from build123d import *

# Parameters (mm, degrees)
SKETCH1_R                  = 34.671
BOSS_EXTRUDE1_DEPTH        = 9.525
FILLET1_R                  = 5.08
SKETCH2_R                  = 4.0005
CUT_EXTRUDE1_DEPTH         = 5.08
F_10_CLEARANCE_HOLE1_D     = 5.1054
F_10_CLEARANCE_HOLE1_DEPTH = 4.445


with BuildPart() as part:
    # Sketch1 → Boss-Extrude1 (new body)
    with BuildSketch(Plane.XY):
        with Locations(Location((0, 0, 0), (0, 0, 180))):
            Circle(SKETCH1_R)
        with BuildLine():
            ThreePointArc((19.058413969, -22.135965238), (29.21, 0), (19.058413969, 22.135965238))
            ThreePointArc((19.058413969, 22.135965238), (11.8745, 20.567237314), (9.641101249, 27.573053271))
            ThreePointArc((9.641101249, 27.573053271), (-14.605, 25.296602045), (-28.699515217, 5.437088034))
            ThreePointArc((-28.699515217, 5.437088034), (-23.749, 0), (-28.699515217, -5.437088034))
            ThreePointArc((-28.699515217, -5.437088034), (-14.605, -25.296602045), (9.641101249, -27.573053271))
            ThreePointArc((9.641101249, -27.573053271), (11.8745, -20.567237314), (19.058413969, -22.135965238))
        make_face(mode=Mode.SUBTRACT)
    extrude(amount=BOSS_EXTRUDE1_DEPTH)

    # Fillet1
    fillet1_edges = [part.edges().sort_by_distance(p)[0] for p in [
        (-28.699515217, 5.437088034, 4.7625),
        (-28.699515217, -5.437088034, 4.7625),
        (9.641101249, -27.573053271, 4.7625),
        (19.058413969, -22.135965238, 4.7625),
        (19.058413969, 22.135965238, 4.7625),
        (9.641101249, 27.573053271, 4.7625),
    ]]
    fillet(fillet1_edges, radius=FILLET1_R)

    # Sketch2 → Cut-Extrude1 (cut)
    with BuildSketch(Plane(origin=(0, 0, 0), x_dir=(-1, 0, 0), z_dir=(0, 0, -1))):
        with Locations((-14.605, 25.296602045)):
            Circle(SKETCH2_R)
        with Locations((29.21, 0)):
            Circle(SKETCH2_R)
        with Locations((-14.605, -25.296602045)):
            Circle(SKETCH2_R)
    extrude(amount=-CUT_EXTRUDE1_DEPTH, mode=Mode.SUBTRACT)

    # #10 Clearance Hole1
    with Locations(Plane(origin=(0, 0, 5.08), x_dir=(-1, 0, 0), z_dir=(0, 0, -1))):
        with Locations((-14.605, 25.296602045), (29.21, 0), (-14.605, -25.296602045), (0, 0)):
            Hole(F_10_CLEARANCE_HOLE1_D / 2, depth=F_10_CLEARANCE_HOLE1_DEPTH)


solid = part.part
Work out the finished part from the listing and answer in its coordinate system (mm). A direction names the side the tool comes from. Coordinates: 2 decimals unless noted, no trailing zeros. Write each loop counter-clockwise with the first axis right and the second up, starting at its lowest first coordinate (ties: lowest second). Pieces come first, ordered by that corner, then holes. Notation, with made-up numbers: M 75,16 L 131,16 A21 cw 131,24 Z; hole C 55,11.25 d7. An arc over 180 degrees is marked long. Use one line per item in the form item = value. Start each with the question number.
1. The part is cut by section C-C (x = -17). Give the vertices of the cut face in (y, z) (3 decimals), plus the area to 3 significant figures.
2. The mould has two halves that part along X. Classify faces 1 (the face through (34.637, -1.524, 4.696)), 2 (the face through (13, -21, 9.525)), 3 (the face through (-26.035, -2.434, 2.504)): released by +X, released by -X, zero draft, split by the parting line, or undercut.
3. A tool of negligible diameter and unlimited length cuts with its end or side. For faces 4 (the face through (15.472, -29.202, 2.504)), 5 (the face through (11.934, 20.533, 4.696)), 6 (the face through (13, 20.4, 0)), from which of +Z, -Z, +X, -X, +Y, -Y can it reach the whole face along a straight path? Write none if from no direction.
4. The part is cut by section A-A (y = 0). Give the vertices of the cut face in (x, z) (1 decimal).
5. Each of these flat-tipped pins is pushed along its axis until it touches: P1, Ø4, axis at y = 13, z = 6.5, coming from the +X side; P2, Ø1.5, axis at x = -11.5, z = 2, coming from the +Y side; P3, Ø1.5, axis at x = 26, y = 6.5, coming from the -Z side; P4, Ø5, axis at x = 22, z = 5, coming from the -Y side. Where does it stop, or does it pass through?
6. The part is cut by section B-B (x = 0). Give the vertices of the cut face in (y, z) (3 decimals).
7. The part is cut by section D-D (z = 3.25). Give the number of separate pieces and of enclosed holes in the cut face, plus the area to 3 significant figures.
8. Straight lines are drawn through the part: probe 1 along Y at (x, z) = (-24.5, 4.5); probe 2 along X at (y, z) = (-15.5, 2.75); probe 3 along X at (y, z) = (-10.5, 8.5). For each, find the intervals that lie inside material, in ascending order. Write a range as from..to.
Evaluation:
q1.outline = M -30.217,0 L -23.753,0 L -23.753,9.525 L -30.217,9.525 Z; M 23.753,0 L 30.217,0 L 30.217,9.525 L 23.753,9.525 Z
q1.area = 123 mm^2
q2.face_1 = split by the parting line
q2.face_2 = zero draft
q2.face_3 = undercut
q3.face_4 = -Z
q3.face_5 = +Z, -Z
q3.face_6 = -Z, +X, -X, +Y, -Y
q4.outline = M -34.7,0 L -33.2,0 L -33.2,5.1 L -31.8,5.1 L -31.8,9.5 L -34.7,9.5 Z; M -26.7,5.1 L -25.2,5.1 L -25.2,0 L -23.7,0 L -23.7,9.5 L -26.7,9.5 Z; M 29.2,0 L 34.7,0 L 34.7,9.5 L 29.2,9.5 Z
q5.P1 = 32.88
q5.P2 = 32.96
q5.P3 = through
q5.P4 = -28.67
q6.outline = M -34.671,0 L -29.21,0 L -29.21,9.525 L -34.671,9.525 Z; M 29.21,0 L 34.671,0 L 34.671,9.525 L 29.21,9.525 Z
q7.separate_pieces = 1
q7.enclosed_holes = 4
q7.area = 1,100 mm^2
q8.probe_1 = -24.53..-15.91, -2.76..2.76, 15.91..24.53
q8.probe_2 = -31.01..-24.76, 24.76..31.01
q8.probe_3 = -33.04..-27.26, 27.26..33.04
